```python
from build123d import *

# Parameters (mm, degrees)
SKETCH1_W            = 25
SKETCH1_H            = 25
BOSS_EXTRUDE1_DEPTH  = 2
SKETCH2_R            = 0.8
CUT_EXTRUDE1_DEPTH   = 18.790446875
LPATTERN1_COUNT      = 2
LPATTERN1_PITCH      = 20
LPATTERN1_COUNT_DIR2 = 2
LPATTERN1_PITCH_DIR2 = 13
SKETCH3_R            = 1.6
BOSS_EXTRUDE2_DEPTH  = 6.9
FILLET1_R            = 1


with BuildPart() as part:
    # Sketch1 → Boss-Extrude1 (new body)
    with BuildSketch(Plane.XY):
        Rectangle(SKETCH1_W, SKETCH1_H)
    extrude(amount=BOSS_EXTRUDE1_DEPTH)

    # Sketch2 → Cut-Extrude1 (cut, through all)
    with BuildSketch(Plane.XY.offset(2)):
        with Locations((-10, 10)):
            Circle(SKETCH2_R)
    cut_extrude1 = extrude(amount=-CUT_EXTRUDE1_DEPTH, mode=Mode.SUBTRACT)

    # LPattern1: Cut-Extrude1 2 × 2
    with Locations(*[(i * LPATTERN1_PITCH, -j * LPATTERN1_PITCH_DIR2, 0) for i in range(LPATTERN1_COUNT) for j in range(LPATTERN1_COUNT_DIR2) if (i, j) != (0, 0)]):
        add(cut_extrude1, mode=Mode.SUBTRACT)

    # Sketch3 → Boss-Extrude2 (add)
    with BuildSketch(Plane(origin=(0, 0, 0), x_dir=(1, 0, 0), z_dir=(0, 1, 0))):
        with BuildLine():
            Line((12.5, 0), (-5.42402052, 0))
            Line((-5.42402052, 0), (0.684667897, 24.049376833))
            ThreePointArc((0.684667897, 24.049376833), (7.244314241, 28.525901035), (12.5, 22.572247005))
            Line((12.5, 22.572247005), (12.5, 0))
        make_face()
        with Locations(Location((6.5, 22.572247005, 0), (0, 0, 90))):
            Circle(SKETCH3_R, mode=Mode.SUBTRACT)
        with BuildLine():
            Line((1.361051754, 3.446753303), (7.227967943, 3.446753303))
            ThreePointArc((7.227967943, 3.446753303), (7.935074725, 3.739646522), (8.227967943, 4.446753303))
            Line((8.227967943, 4.446753303), (8.227967943, 12.628736978))
            ThreePointArc((8.227967943, 12.628736978), (5.718628608, 15.471322881), (2.586710272, 13.333996035))
            Line((2.586710272, 13.333996035), (0.391829737, 4.692941607))
            ThreePointArc((0.391829737, 4.692941607), (0.571688623, 3.832826721), (1.361051754, 3.446753303))
        make_face(mode=Mode.SUBTRACT)
    extrude(amount=BOSS_EXTRUDE2_DEPTH)

    # Fillet1
    fillet1_edges = [part.edges().sort_by_distance(p)[0] for p in [
        (12.5, 6.9, -11.286123503),
        (7.244314241, 6.9, -28.525901035),
        (-2.369676312, 6.9, -12.024688416),
        (8.227967943, 0, -8.53774514),
        (5.718628608, 0, -15.471322881),
        (1.489270004, 0, -9.013468821),
        (0.571688623, 0, -3.832826721),
        (4.294509849, 0, -3.446753303),
        (7.935074725, 0, -3.739646522),
        (12.5, 0, -11.286123503),
        (7.244314241, 0, -28.525901035),
        (-2.369676312, 0, -12.024688416),
        (5.718628608, 6.9, -15.471322881),
        (1.489270004, 6.9, -9.013468821),
        (0.571688623, 6.9, -3.832826721),
        (4.294509849, 6.9, -3.446753303),
        (7.935074725, 6.9, -3.739646522),
        (8.227967943, 6.9, -8.53774514),
        (12.5, -12.5, 1),
        (-12.5, -12.5, 1),
        (-12.5, 12.5, 1),
        (12.5, 12.5, 1),
    ]]
    fillet(fillet1_edges, radius=FILLET1_R)


solid = part.part
```
For this review, take the finished solid that the model builds, in its own axes (mm). A direction names the side the tool comes from. Give positions to 0.01 mm unless a question says otherwise; leave off trailing zeros. Write each loop counter-clockwise with the first axis right and the second up, starting at its lowest first coordinate (ties: lowest second). Pieces come first, ordered by that corner, then holes.
Item 1: Take a section at A-A (y = 10). Give the boundary of the cut face in (x, z), and give its area (3 significant figures).
Item 2: The part is to be moulded in two halves that separate along X. For faces 1 (the face through (-12.215, 12.199, 1.014)), 2 (the face through (0, -12.5, 1)), 3 (the face through (12.215, 0.301, -11.128)), 4 (the face through (-10.104, 10.793, 1.014)), say which applies: +X half, -X half, draft (parallel to the pull), parting line (faces both ways), or undercut.
Item 3: Insertion check: P1, Ø1.5, axis at y = 2.5, z = -7, coming from the -X side; P2, Ø2, axis at x = 2, y = 8, coming from the -Z side; P3, Ø1.5, axis at x = 1, z = -9.5, coming from the -Y side. Each pin has a flat end and moves straight along its axis. Give the tip position at first contact, or say it passes through.
Item 4: Take a section at C-C (y = 2.5). Give the boundary of the cut face in (x, z).
Item 5: Take a section at B-B (x = -10). Give the boundary of the cut face in (y, z).
Item 6: Take a section at D-D (y = -5). Give the boundary of the cut face in (x, z), and give its area (3 significant figures).
Item 7: Machinability: for faces 5 (the face through (5, 6.9, -17)), 6 (the face through (5, 0, -17)), 7 (the face through (4.34, 6.61, -3.15)), 8 (the face through (4.34, 0.29, -3.15)), 9 (the face through (8.228, 3, -8)), which of the approach directions +Z, -Z, +X, -X, +Y, -Y give a long, thin tool a straight path to every point of the face, cutting with its end or side? Answer none if there is none.
Item 8: Wall thickness on probe 1 along Y at (x, z) = (-10, 0.55); probe 2 along Z at (x, y) = (5.5, 2.25); probe 3 along Z at (x, y) = (-11, 2): over which ranges is each line inside the solid? List them lowest first.
Established:
1. outline: (-12.5, 0) - (-10.8, 0) - (-10.8, 2) - (-12.5, 2) - close; (-9.2, 0) - (9.2, 0) - (9.2, 2) - (-9.2, 2) - close; (10.8, 0) - (12.5, 0) - (12.5, 2) - (10.8, 2) - close
1. area: 43.6 mm2
2. face 1: -X half
2. face 2: draft
2. face 3: +X half
2. face 4: undercut
3. P1: stops at x = -3.84
3. P2: stops at z = 0
3. P3: stops at y = 0
4. outline: (-12.5, 0) - (-5.42, 0) - (0.68, -24.05) arc R6 ccw to (12.5, -22.57) - (12.5, 2) - (-12.5, 2) - close; hole (0.39, -4.69) - (2.59, -13.33) arc R2.86 ccw to (8.23, -12.63) - (8.23, -4.45) arc R1 ccw to (7.23, -3.45) - (1.36, -3.45) arc R1 ccw to start; hole circle Ø3.2 at (6.5, -22.57)
5. outline: (-12.5, 0) - (-3.8, 0) - (-3.8, 2) - (-12.5, 2) - close; (-2.2, 0) - (9.2, 0) - (9.2, 2) - (-2.2, 2) - close; (10.8, 0) - (12.5, 0) - (12.5, 2) - (10.8, 2) - close
6. outline: (-12.5, 0) - (12.5, 0) - (12.5, 2) - (-12.5, 2) - close
6. area: 50.0 mm2
7. face 5: -Z, +X, -X, +Y
7. face 6: -Z, +X, -X, -Y
7. face 7: +Y
7. face 8: -Y
7. face 9: +Y, -Y
8. probe 1: y = -12.5 to -3.8, -2.2 to 9.2, 10.8 to 12.5
8. probe 2: z = -28.49 to -23.82, -21.32 to -15.49, -3.45 to 2
8. probe 3: z = 0 to 2
